CAD build for the part. Positions are in the model's coordinates, mm. A direction names the side the tool comes from. Give positions to 0.01 mm unless a question says otherwise; leave off trailing zeros. Loops run counter-clockwise (first coordinate to the right, second up) from the corner with the lowest first, then second, coordinate; pieces in that order, holes last.
```python
from build123d import *

# Parameters (mm, degrees)
SKETCH1_R                       = 2.5
BOSS_EXTRUDE1_DEPTH             = 21.21
SKETCH2_R                       = 11
BOSS_EXTRUDE2_DEPTH             = 2.4
SKETCH3_W                       = 42.418
SKETCH3_H                       = 42.418
BOSS_EXTRUDE3_DEPTH             = 39.24
CUT_EXTRUDE1_DEPTH              = 61.45
M3X0_5_TAPPED_HOLE1_D           = 2.5
M3X0_5_TAPPED_HOLE1_DEPTH       = 7.5
M3X0_5_TAPPED_HOLE1_CBORE_D     = 3
M3X0_5_TAPPED_HOLE1_CBORE_DEPTH = 6
M3X0_5_TAPPED_HOLE1_TIP         = 0.751075774
CUT_EXTRUDE2_DEPTH              = 15
CUT_EXTRUDE3_DEPTH              = 10.87


with BuildPart() as part:
    # Sketch1 → Boss-Extrude1 (new body)
    with BuildSketch(Plane.XY):
        Circle(SKETCH1_R)
    extrude(amount=BOSS_EXTRUDE1_DEPTH)

    # Sketch2 → Boss-Extrude2 (add)
    with BuildSketch(Plane(origin=(0, 0, 0), x_dir=(-1, 0, 0), z_dir=(0, 0, -1))):
        Circle(SKETCH2_R)
    extrude(amount=-BOSS_EXTRUDE2_DEPTH)

    # Sketch3 → Boss-Extrude3 (add)
    with BuildSketch(Plane(origin=(0, 0, 0), x_dir=(-1, 0, 0), z_dir=(0, 0, -1))):
        Rectangle(SKETCH3_W, SKETCH3_H)
    extrude(amount=BOSS_EXTRUDE3_DEPTH)

    # Sketch4 → Cut-Extrude1 (cut, through all)
    with BuildSketch(Plane(origin=(0, 0, -39.24), x_dir=(-1, 0, 0), z_dir=(0, 0, -1))):
        with BuildLine():
            Line((-21.209, -15.887992919), (-21.209, -21.209))
            Line((-21.209, -21.209), (-15.887992919, -21.209))
            ThreePointArc((-15.887992919, -21.209), (-18.738329701, -18.738329701), (-21.209, -15.887992919))
        make_face()
        with BuildLine():
            Line((15.887992919, -21.209), (21.209, -21.209))
            Line((21.209, -21.209), (21.209, -15.887992919))
            ThreePointArc((21.209, -15.887992919), (18.738329701, -18.738329701), (15.887992919, -21.209))
        make_face()
        with BuildLine():
            Line((21.209, 15.887992919), (21.209, 21.209))
            Line((21.209, 21.209), (15.887992919, 21.209))
            ThreePointArc((15.887992919, 21.209), (18.738329701, 18.738329701), (21.209, 15.887992919))
        make_face()
        with BuildLine():
            Line((-15.887992919, 21.209), (-21.209, 21.209))
            Line((-21.209, 21.209), (-21.209, 15.887992919))
            ThreePointArc((-21.209, 15.887992919), (-18.738329701, 18.738329701), (-15.887992919, 21.209))
        make_face()
    extrude(amount=-CUT_EXTRUDE1_DEPTH, mode=Mode.SUBTRACT)

    # M3x0.5 Tapped Hole1
    with Locations(Plane.XY):
        with Locations((-15.5, 15.5), (-15.5, -15.5), (15.5, -15.5), (15.5, 15.5)):
            CounterBoreHole(M3X0_5_TAPPED_HOLE1_D / 2, M3X0_5_TAPPED_HOLE1_CBORE_D / 2, M3X0_5_TAPPED_HOLE1_CBORE_DEPTH, depth=M3X0_5_TAPPED_HOLE1_DEPTH)
            with Locations((0, 0, -(M3X0_5_TAPPED_HOLE1_DEPTH + M3X0_5_TAPPED_HOLE1_TIP / 2))):  # 118° drill point
                Cone(0, M3X0_5_TAPPED_HOLE1_D / 2, M3X0_5_TAPPED_HOLE1_TIP, mode=Mode.SUBTRACT)

    # Sketch7 → Cut-Extrude2 (cut)
    with BuildSketch(Plane.XY.offset(21.21)):
        with BuildLine():
            Line((-1.5, 2), (1.5, 2))
            ThreePointArc((1.5, 2), (0, 2.5), (-1.5, 2))
        make_face()
    extrude(amount=-CUT_EXTRUDE2_DEPTH, mode=Mode.SUBTRACT)

    # Sketch8 → Cut-Extrude3 (cut, symmetric)
    with BuildSketch(Plane.XY.offset(-19.62)):
        with BuildLine():
            Line((15.887992919, 21.209), (-15.887992919, 21.209))
            ThreePointArc((-15.887992919, 21.209), (-18.738329701, 18.738329701), (-21.209, 15.887992919))
            Line((-21.209, 15.887992919), (-21.209, -15.887992919))
            ThreePointArc((-21.209, -15.887992919), (-18.738329701, -18.738329701), (-15.887992919, -21.209))
            Line((-15.887992919, -21.209), (15.887992919, -21.209))
            ThreePointArc((15.887992919, -21.209), (18.738329701, -18.738329701), (21.209, -15.887992919))
            Line((21.209, -15.887992919), (21.209, 15.887992919))
            ThreePointArc((21.209, 15.887992919), (18.738329701, 18.738329701), (15.887992919, 21.209))
        make_face()
        with BuildLine():
            Line((-13.394406258, 21.109), (13.394406258, 21.109))
            ThreePointArc((13.394406258, 21.109), (17.67766953, 17.67766953), (21.109, 13.394406258))
            Line((21.109, 13.394406258), (21.109, -13.394406258))
            ThreePointArc((21.109, -13.394406258), (17.67766953, -17.67766953), (13.394406258, -21.109))
            Line((13.394406258, -21.109), (-13.394406258, -21.109))
            ThreePointArc((-13.394406258, -21.109), (-17.67766953, -17.67766953), (-21.109, -13.394406258))
            Line((-21.109, -13.394406258), (-21.109, 13.394406258))
            ThreePointArc((-21.109, 13.394406258), (-17.67766953, 17.67766953), (-13.394406258, 21.109))
        make_face(mode=Mode.SUBTRACT)
    extrude(amount=CUT_EXTRUDE3_DEPTH, both=True, mode=Mode.SUBTRACT)


solid = part.part
```
1. Tool access for faces 4 (the face through (0, -21.109, -19)), 5 (the face through (-19, 17, -8.75)), 6 (the face through (-21.109, 0, -19)), 7 (the face through (0, 2, 14)), 8 (the face through (-15.34, -14.26, -6.76)): list every direction of +Z, -Z, +X, -X, +Y, -Y with a clear straight run to the whole face (end or side of a thin tool).
Responses:
face 4: +X, -X, -Y
face 5: none
face 6: -X, +Y, -Y
face 7: +Z, +X, -X, +Y
face 8: +Z
2. Probe line 1 along X through (y, z) = (15.5, -6.9); line 2 along Z through (x, y) = (-15, 10.5). List the from-to ranges inside material, lowest first.
Responses:
line 1: x = -21.21 to -16.75, -14.25 to 14.25, 16.75 to 21.21
line 2: z = -39.24 to 0
3. Pull direction Z, two halves, no side cores. Call faces 1 (the face through (-9, -9, 0)), 2 (the face through (-19, 17, -30.49)), 3 (the face through (16.421, 16.345, -6.76)): released by +Z, released by -Z, zero draft, split by the parting line, or undercut.
Responses:
face 1: released by +Z
face 2: undercut
face 3: zero draft
4. Saw through at C-C, the plane y = 0. List the corners of the cut face in (x, z), and give its area (3 significant figures).
Responses:
outline: (-21.21, -39.24) - (21.21, -39.24) - (21.21, -30.49) - (21.11, -30.49) - (21.11, -8.75) - (21.21, -8.75) - (21.21, 0) - (11, 0) - (11, 2.4) - (2.5, 2.4) - (2.5, 21.21) - (-2.5, 21.21) - (-2.5, 2.4) - (-11, 2.4) - (-11, 0) - (-21.21, 0) - (-21.21, -8.75) - (-21.11, -8.75) - (-21.11, -30.49) - (-21.21, -30.49) - close
area: 1,810 mm2
5. Drop flat-ended pins along their axis: pin 1 (2.5 mm diameter, centred on x = 15, y = 15.5, fed in from +Z); pin 2 (1.5 mm diameter, centred on x = 0, z = 11, fed in from +Y); pin 3 (2 mm diameter, centred on x = -8.5, z = -27.5, fed in from +Y). Give the stop position or say it passes through.
Responses:
pin 1: stops at z = 0
pin 2: stops at y = 2
pin 3: stops at y = 21.11
6. Saw through at B-B, the plane z = -19. List the corners of the cut face in (x, y).
Responses:
outline: (-21.11, -13.39) arc R25 ccw to (-13.39, -21.11) - (13.39, -21.11) arc R25 ccw to (21.11, -13.39) - (21.11, 13.39) arc R25 ccw to (13.39, 21.11) - (-13.39, 21.11) arc R25 ccw to (-21.11, 13.39) - close
7. Saw through at D-D, the plane x = -10. List the corners of the cut face in (y, z), and give its area (3 significant figures).
Responses:
outline: (-21.21, -39.24) - (21.21, -39.24) - (21.21, -30.49) - (21.11, -30.49) - (21.11, -8.75) - (21.21, -8.75) - (21.21, 0) - (4.58, 0) - (4.58, 2.4) - (-4.58, 2.4) - (-4.58, 0) - (-21.21, 0) - (-21.21, -8.75) - (-21.11, -8.75) - (-21.11, -30.49) - (-21.21, -30.49) - close
area: 1,680 mm2
8. Saw through at A-A, the plane x = 0. List the corners of the cut face in (y, z).
Responses:
outline: (-21.21, -39.24) - (21.21, -39.24) - (21.21, -30.49) - (21.11, -30.49) - (21.11, -8.75) - (21.21, -8.75) - (21.21, 0) - (11, 0) - (11, 2.4) - (2.5, 2.4) - (2.5, 6.21) - (2, 6.21) - (2, 21.21) - (-2.5, 21.21) - (-2.5, 2.4) - (-11, 2.4) - (-11, 0) - (-21.21, 0) - (-21.21, -8.75) - (-21.11, -8.75) - (-21.11, -30.49) - (-21.21, -30.49) - close
